Source: CAD feature listing. Evaluate the final solid. Frame: model axes, mm. A direction names the side the tool comes from. Round coordinates to 2 decimals unless told otherwise and drop trailing zeros. Loops run counter-clockwise (first coordinate to the right, second up) from the corner with the lowest first, then second, coordinate; pieces in that order, holes last. Notation, with made-up numbers: M -19,-6 L 39,-6 A20 ccw 39,31 Z; hole C 31.5,45.25 d1. An arc over 180 degrees is marked long. One line per item, written item: value.
from build123d import *

# Parameters (mm, degrees)
SKETCH3_R           = 4
CUT_EXTRUDE5_DEPTH  = 10
CIRPATTERN1_COUNT   = 6
SKETCH4_R           = 23.5
CUT_EXTRUDE6_DEPTH  = 90
SKETCH5_W           = 16
SKETCH5_H           = 16
BOSS_EXTRUDE1_START = -16
SKETCH6_W           = 2
SKETCH6_H           = 2.4
BOSS_EXTRUDE1_DEPTH = 16
CIRPATTERN2_COUNT   = 12
SKETCH7_R           = 31
SKETCH7_R_2         = 30
CUT_EXTRUDE7_DEPTH  = 32.87


with BuildPart() as part:
    # Sketch1 → Revolve1 (revolve)
    with BuildSketch(Plane.XY):
        Polygon((0, 0), (0, 31), (7, 31), (7, 44), (16.5, 44), (19.87, 40.63), (19.87, 31), (118.87, 31), (118.87, 0), align=None)
    revolve(axis=Axis((118.87, 0, 0), (-1, 0, 0)))

    # Sketch3 → Cut-Extrude5 (cut)
    with BuildSketch(Plane.ZY.offset(-7)):
        with Locations(Location((0, 37.5, 0), (0, 0, 270))):
            Circle(SKETCH3_R)
    cut_extrude5 = extrude(amount=-CUT_EXTRUDE5_DEPTH, mode=Mode.SUBTRACT)

    # CirPattern1: Cut-Extrude5 ×6 about axis
    cirpattern1_axis = Axis((0, 0, 0), (1, 0, 0))
    for i in range(1, CIRPATTERN1_COUNT):
        add(cut_extrude5.rotate(cirpattern1_axis, i * 360 / CIRPATTERN1_COUNT), mode=Mode.SUBTRACT)

    # Sketch4 → Cut-Extrude6 (cut)
    with BuildSketch(Plane.ZY):
        with Locations(Location((0, 0, 0), (0, 0, 270))):
            Circle(SKETCH4_R)
    extrude(amount=-CUT_EXTRUDE6_DEPTH, mode=Mode.SUBTRACT)

    # Sketch5 → Revolve2 (revolve)
    with BuildSketch(Plane.XY, mode=Mode.PRIVATE) as revolve2_sk:
        with Locations((82, 18)):
            Rectangle(SKETCH5_W, SKETCH5_H)
    revolve(revolve2_sk.sketch.rotate(Axis((118.87, 0, 0), (-1, 0, 0)), 180), axis=Axis((118.87, 0, 0), (-1, 0, 0)))

    # Sketch6 → Boss-Extrude1 (add)
    with BuildSketch(Plane.ZY.offset(-74).offset(BOSS_EXTRUDE1_START)):
        with Locations((0, 9.8)):
            Rectangle(SKETCH6_W, SKETCH6_H)
    boss_extrude1 = extrude(amount=BOSS_EXTRUDE1_DEPTH)

    # CirPattern2: Boss-Extrude1 ×12 about axis
    cirpattern2_axis = Axis((0, 0, 0), (1, 0, 0))
    for i in range(1, CIRPATTERN2_COUNT):
        add(boss_extrude1.rotate(cirpattern2_axis, i * 360 / CIRPATTERN2_COUNT))

    # Sketch7 → Cut-Extrude7 (cut)
    with BuildSketch(Plane(origin=(118.87, 0, 0), x_dir=(0, 0, -1), z_dir=(1, 0, 0))):
        with Locations(Location((0, 0, 0), (0, 0, 90))):
            Circle(SKETCH7_R)
        with Locations(Location((0, 0, 0), (0, 0, 90))):
            Circle(SKETCH7_R_2, mode=Mode.SUBTRACT)
    extrude(amount=-CUT_EXTRUDE7_DEPTH, mode=Mode.SUBTRACT)


solid = part.part
1. Pin query (flat end, axial travel): pin 1 (7 mm diameter, centred on y = 18.75, z = -32.48, fed in from -X); pin 2 (1.5 mm diameter, centred on x = 83, y = -9.5, fed in from -Z); pin 3 (8 mm diameter, centred on y = -13.5, z = 2, fed in from -X). Return the tip coordinate at first contact, or that it passes through.
Report:
pin 1: stops at x = 17
pin 2: stops at z = -29.74
pin 3: stops at x = 74
2. Reachability of faces 4 (the face through (86, -12, 28)), 5 (the face through (11.93, -17.88, 28.57)), 6 (the face through (0, -11, -21)) from +Z, -Z, +X, -X, +Y, -Y: full face, straight path, thin tool, end or side. Return the list, or none.
Report:
face 4: +X
face 5: -X
face 6: +Z, -Z, -X, +Y, -Y
3. Section query B-B (x = 97). Return the cut outline in (y, z).
Report:
outline: C 0,0 d60
4. Ray query, line 1 (Z direction, x = 15.25, y = 18.75) (3 decimals); line 2 (Z direction, x = 7.5, y = 19); line 3 (X direction, y = -2.5, z = -8.5). Return the intervals inside material, ascending. Write a range as [from, to].
Report:
line 1: z = [-39.805, -36.476], [-28.476, -14.166], [14.166, 28.476], [36.476, 39.805]
line 2: z = [-39.69, -36.47], [-28.48, -13.83], [13.83, 28.48], [36.47, 39.69]
line 3: x = [90, 118.87]
5. Section query A-A (x = 40). Return the cut outline in (y, z), and give its area (3 significant figures).
Report:
outline: C 0,0 d62; hole C 0,0 d47
area: 1,280 mm2
6. Pull-direction query (Z, two-part tool) for faces 1 (the face through (53.398, -4.036, -30.736)), 2 (the face through (7, 30, 10)), 3 (the face through (82.112, 9.665, -2.566)); classes: released by +Z, released by -Z, zero draft, split by the parting line, or undercut.
Report:
face 1: split by the parting line
face 2: zero draft
face 3: undercut
